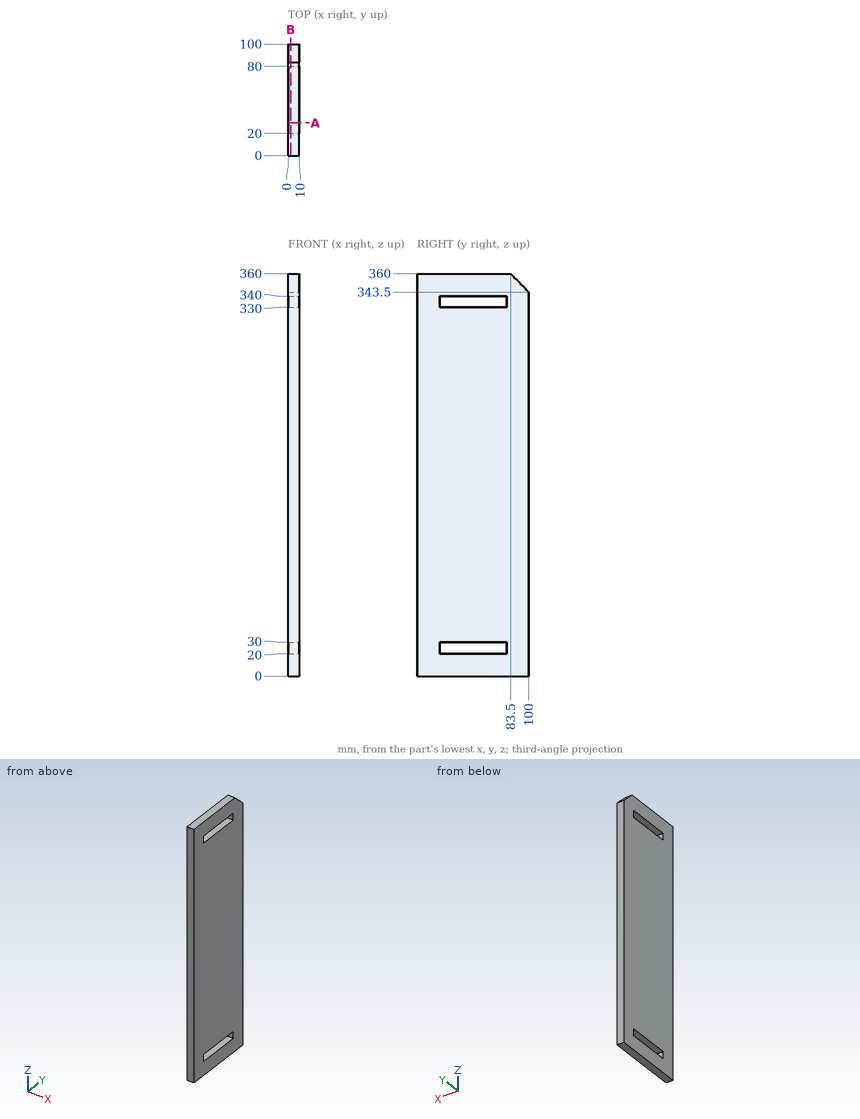
Verification items for this drawing (mm, ordinates from the low corner). Give positions to 0.01 mm unless a question says otherwise; leave off trailing zeros. Write each loop counter-clockwise with the first axis right and the second up, starting at its lowest first coordinate (ties: lowest second). Pieces come first, ordered by that corner, then holes. Notation, with made-up numbers: (20, 50.25) - (77, 50.25) arc R28 ccw to (77, 80.25) - close; hole circle Ø6 at (-15.75, 38). An arc over 180 degrees is marked (long way). Answer as CSV lines item,"result". Start each with the question number.
1. Thickness scan on line 1 (Z direction, x = 2, y = 42); line 2 (Y direction, x = 9.25, z = 336); line 3 (Z direction, x = 4.5, y = 95). Record the ranges inside material, lowest first.
2. Sectioned sample at A-A (y = 29.5). Record the boundary of the cut face in (x, z), then the cut area to 3 significant figures.
3. Sectioned sample at B-B (x = 2.25). Record the boundary of the cut face in (y, z).
Derived:
1,line 1,"0 to 20, 30 to 330, 340 to 360"
1,line 2,"0 to 20, 80 to 100"
1,line 3,"0 to 348.5"
2,outline,"(0, 0) - (10, 0) - (10, 20) - (0, 20) - close; (0, 30) - (10, 30) - (10, 330) - (0, 330) - close; (0, 340) - (10, 340) - (10, 360) - (0, 360) - close"
2,area,"3,400 mm²"
3,outline,"(0, 0) - (100, 0) - (100, 343.5) - (83.5, 360) - (0, 360) - close; hole (20, 20) - (80, 20) - (80, 30) - (20, 30) - close; hole (20, 330) - (80, 330) - (80, 340) - (20, 340) - close"
